from build123d import *

# Parameters (mm, degrees)
BOTTOM_PLATE_OUTLINE_W   = 160
BOTTOM_PLATE_OUTLINE_H   = 110
BOTTOM_PLATE_OUTLINE_R   = 1.6
BOTTOM_PLATE_OUTLINE_W_2 = 2.95
BOTTOM_PLATE_OUTLINE_H_2 = 10
BOTTOM_PLATE_OUTLINE_W_3 = 10
BOTTOM_PLATE_OUTLINE_H_3 = 2.95
BOTTOM_PLATE_DEPTH       = 2.95
M3_CLEARANCE_HOLE1_D     = 3.2
SKETCH6_W                = 5
SKETCH6_H                = 53.34
CUT_EXTRUDE1_DEPTH       = 98.127249009
FILLET1_R                = 2.5
FILLET2_R                = 2.5
M3_CLEARANCE_HOLE2_D     = 3.2
M3_CLEARANCE_HOLE3_D     = 3.2
SKETCH12_W               = 2.95
SKETCH12_H               = 10
CUT_EXTRUDE4_DEPTH       = 98.127249009


# Read off the part's stored shape, not the designer's step: Bottom Plate
with BuildPart() as part:
    # Bottom Plate outline → Bottom Plate (new body)
    with BuildSketch(Plane(origin=(0, 0, 0), x_dir=(1, 0, 0), z_dir=(0, 1, 0))):
        Rectangle(BOTTOM_PLATE_OUTLINE_W, BOTTOM_PLATE_OUTLINE_H)
        with Locations((-73.525, -48.875)):
            Circle(BOTTOM_PLATE_OUTLINE_R, mode=Mode.SUBTRACT)
        with Locations((-73.525, -30)):
            Rectangle(BOTTOM_PLATE_OUTLINE_W_2, BOTTOM_PLATE_OUTLINE_H_2, mode=Mode.SUBTRACT)
        with Locations((-53.75, -34.729)):
            Rectangle(BOTTOM_PLATE_OUTLINE_W_3, BOTTOM_PLATE_OUTLINE_H_3, mode=Mode.SUBTRACT)
        with Locations((-33.75, -34.729)):
            Rectangle(BOTTOM_PLATE_OUTLINE_W_3, BOTTOM_PLATE_OUTLINE_H_3, mode=Mode.SUBTRACT)
        with Locations((-73.525, -10)):
            Rectangle(BOTTOM_PLATE_OUTLINE_W_2, BOTTOM_PLATE_OUTLINE_H_2, mode=Mode.SUBTRACT)
        with Locations((33.75, -34.729)):
            Rectangle(BOTTOM_PLATE_OUTLINE_W_3, BOTTOM_PLATE_OUTLINE_H_3, mode=Mode.SUBTRACT)
        with Locations((73.525, -48.875)):
            Circle(BOTTOM_PLATE_OUTLINE_R, mode=Mode.SUBTRACT)
        with Locations((53.75, -34.729)):
            Rectangle(BOTTOM_PLATE_OUTLINE_W_3, BOTTOM_PLATE_OUTLINE_H_3, mode=Mode.SUBTRACT)
        with Locations((73.525, -30)):
            Rectangle(BOTTOM_PLATE_OUTLINE_W_2, BOTTOM_PLATE_OUTLINE_H_2, mode=Mode.SUBTRACT)
        with Locations((73.525, -10)):
            Rectangle(BOTTOM_PLATE_OUTLINE_W_2, BOTTOM_PLATE_OUTLINE_H_2, mode=Mode.SUBTRACT)
        with Locations((-73.525, 10)):
            Rectangle(BOTTOM_PLATE_OUTLINE_W_2, BOTTOM_PLATE_OUTLINE_H_2, mode=Mode.SUBTRACT)
        with Locations((-73.525, 30)):
            Rectangle(BOTTOM_PLATE_OUTLINE_W_2, BOTTOM_PLATE_OUTLINE_H_2, mode=Mode.SUBTRACT)
        with Locations((-53.75, 34.729)):
            Rectangle(BOTTOM_PLATE_OUTLINE_W_3, BOTTOM_PLATE_OUTLINE_H_3, mode=Mode.SUBTRACT)
        with Locations((-73.525, 48.875)):
            Circle(BOTTOM_PLATE_OUTLINE_R, mode=Mode.SUBTRACT)
        with Locations((-33.75, 34.729)):
            Rectangle(BOTTOM_PLATE_OUTLINE_W_3, BOTTOM_PLATE_OUTLINE_H_3, mode=Mode.SUBTRACT)
        with Locations((73.525, 10)):
            Rectangle(BOTTOM_PLATE_OUTLINE_W_2, BOTTOM_PLATE_OUTLINE_H_2, mode=Mode.SUBTRACT)
        with Locations((33.75, 34.729)):
            Rectangle(BOTTOM_PLATE_OUTLINE_W_3, BOTTOM_PLATE_OUTLINE_H_3, mode=Mode.SUBTRACT)
        with Locations((53.75, 34.729)):
            Rectangle(BOTTOM_PLATE_OUTLINE_W_3, BOTTOM_PLATE_OUTLINE_H_3, mode=Mode.SUBTRACT)
        with Locations((73.525, 30)):
            Rectangle(BOTTOM_PLATE_OUTLINE_W_2, BOTTOM_PLATE_OUTLINE_H_2, mode=Mode.SUBTRACT)
        with Locations((73.525, 48.875)):
            Circle(BOTTOM_PLATE_OUTLINE_R, mode=Mode.SUBTRACT)
    extrude(amount=BOTTOM_PLATE_DEPTH)

    # M3 Clearance Hole1 (through all)
    with Locations(Plane(origin=(0, 2.95, 0), x_dir=(1, 0, 0), z_dir=(0, 1, 0))):
        with Locations((-51.81, 24.13), (-53.08, -24.13), (-1.01, -19.05), (-1.01, 8.89)):
            Hole(M3_CLEARANCE_HOLE1_D / 2)

    # Sketch6 → Cut-Extrude1 (cut, through all)
    with BuildSketch(Plane(origin=(0, 2.95, 0), x_dir=(1, 0, 0), z_dir=(0, 1, 0))):
        with Locations((9.03, 0)):
            Rectangle(SKETCH6_W, SKETCH6_H)
    extrude(amount=-CUT_EXTRUDE1_DEPTH, mode=Mode.SUBTRACT)

    # Fillet1
    fillet1_edges = [part.edges().sort_by_distance(p)[0] for p in [
        (6.53, 1.475, -26.67),
        (11.53, 1.475, -26.67),
    ]]
    fillet(fillet1_edges, radius=FILLET1_R - 0.0001)  # a hair under: the kernel refuses the full size

    # Fillet2
    fillet2_edges = [part.edges().sort_by_distance(p)[0] for p in [
        (6.53, 1.475, 26.67),
        (11.53, 1.475, 26.67),
    ]]
    fillet(fillet2_edges, radius=FILLET2_R - 0.0001)  # a hair under: the kernel refuses the full size

    # M3 Clearance Hole2 (through all)
    with Locations(Plane(origin=(0, 2.95, 0), x_dir=(1, 0, 0), z_dir=(0, 1, 0))):
        with Locations((73.525, -20), (73.525, 20)):
            Hole(M3_CLEARANCE_HOLE2_D / 2)

    # M3 Clearance Hole3 (through all)
    with Locations(Plane(origin=(0, 2.95, 0), x_dir=(1, 0, 0), z_dir=(0, 1, 0))):
        with Locations((9.03, -48.875), (9.03, 48.875)):
            Hole(M3_CLEARANCE_HOLE3_D / 2)

    # Sketch12 → Cut-Extrude4 (cut, through all)
    with BuildSketch(Plane.XZ):
        with Locations((47.275, 10)):
            Rectangle(SKETCH12_W, SKETCH12_H)
        with Locations((47.275, -10)):
            Rectangle(SKETCH12_W, SKETCH12_H)
    cut_extrude4 = extrude(amount=-CUT_EXTRUDE4_DEPTH, mode=Mode.SUBTRACT)

    # Mirror1: Cut-Extrude4 across plane
    add(cut_extrude4.mirror(Plane(origin=(0, 0, 0), x_dir=(0, 0, 1), z_dir=(1, 0, 0))), mode=Mode.SUBTRACT)


solid = part.part
Geometry check sheet. Reference: the model listing, model coordinates, mm. Give positions to 0.01 mm unless a question says otherwise; leave off trailing zeros. Loops run counter-clockwise (first coordinate to the right, second up) from the corner with the lowest first, then second, coordinate; pieces in that order, holes last. Notation, with made-up numbers: (66.25, -11) -> (123.25, -11) arc R15 cw to (123.25, 0) -> close; hole circle Ø2 at (11.5, 76). An arc over 180 degrees is marked (long way). Answer in a Markdown table with one row per item. Add a question column.
1) Cross-section at B-B on x = 31. Record the boundary of the cut face in (y, z).
2) Cross-section at A-A on z = -20. Record the boundary of the cut face in (x, y) (3 decimals), and give its area (3 significant figures).
3) Draft check along Z on faces 1 (the face through (-1, 2.95, -1)), 2 (the face through (6.53, 1, 0)). Enter one of: pulls with the +Z half, pulls with the -Z half, needs draft (parallel to the pull), parting line crosses it, or undercut.
4) Cross-section at D-D on y = 1.5. State how many separate pieces and enclosed holes the cut face has, and give its area (3 significant figures).
5) Cross-section at C-C on z = -8.89. Record the boundary of the cut face in (x, y).
6) Material ranges on probe 1 along Z at (x, y) = (9.03, 2) (3 decimals); probe 2 along X at (y, z) = (1.85, 24.13); probe 3 along Z at (x, y) = (-1.01, 2.45), recorded low to high. Write a range as from..to.
Outcome:
| question | item | result |
|---|---|---|
| 1 | outline | (0, -55) -> (2.95, -55) -> (2.95, -36.2) -> (0, -36.2) -> close; (0, -33.25) -> (2.95, -33.25) -> (2.95, 33.25) -> (0, 33.25) -> close; (0, 36.2) -> (2.95, 36.2) -> (2.95, 55) -> (0, 55) -> close |
| 2 | outline | (-80, 0) -> (6.53, 0) -> (6.53, 2.95) -> (-80, 2.95) -> close; (11.53, 0) -> (71.925, 0) -> (71.925, 2.95) -> (11.53, 2.95) -> close; (75.125, 0) -> (80, 0) -> (80, 2.95) -> (75.125, 2.95) -> close |
| 2 | area | 448 mm^2 |
| 3 | face 1 | needs draft |
| 3 | face 2 | undercut |
| 4 | separate pieces | 1 |
| 4 | enclosed holes | 33 |
| 4 | area | 16,700 mm^2 |
| 5 | outline | (-80, 0) -> (-75, 0) -> (-75, 2.95) -> (-80, 2.95) -> close; (-72.05, 0) -> (-48.75, 0) -> (-48.75, 2.95) -> (-72.05, 2.95) -> close; (-45.8, 0) -> (-2.61, 0) -> (-2.61, 2.95) -> (-45.8, 2.95) -> close; (0.59, 0) -> (6.53, 0) -> (6.53, 2.95) -> (0.59, 2.95) -> close; (11.53, 0) -> (45.8, 0) -> (45.8, 2.95) -> (11.53, 2.95) -> close; (48.75, 0) -> (72.05, 0) -> (72.05, 2.95) -> (48.75, 2.95) -> close; (75, 0) -> (80, 0) -> (80, 2.95) -> (75, 2.95) -> close |
| 6 | probe 1 | z = -55..-50.475, -47.275..-26.67, 26.67..47.275, 50.475..55 |
| 6 | probe 2 | x = -80..-54.68, -51.48..6.53, 11.53..80 |
| 6 | probe 3 | z = -55..-10.49, -7.29..17.45, 20.65..55 |
